Check sheet for the modelled part. Datum: model origin and axes. Units: mm. Face numbers are marked on the shaded views. A direction names the side the tool comes from. Round coordinates to 2 decimals unless told otherwise and drop trailing zeros. Write each loop counter-clockwise with the first axis right and the second up, starting at its lowest first coordinate (ties: lowest second). Pieces come first, ordered by that corner, then holes. Notation, with made-up numbers: (25, 56.5) -> (51, 56.5) arc R11 cw to (51, 60.5) -> close; hole circle Ø8 at (87, -11). An arc over 180 degrees is marked (long way). Write item = value, one per line.
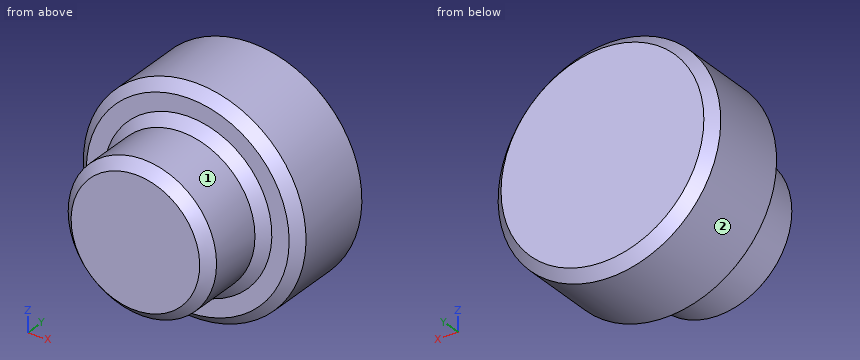
from build123d import *

# Parameters (mm, degrees)
SKETCH_1_R      = 3
EXTRUDE_1_DEPTH = 3
SKETCH_2_R      = 4.5
EXTRUDE_2_DEPTH = 4
CHAMFER_1_SIZE  = 0.4


with BuildPart() as part:
    # 草图1 → 凸台-拉伸1 (new body)
    with BuildSketch(Plane(origin=(0, 0, 0), x_dir=(1, 0, 0), z_dir=(0, 1, 0))):
        with Locations(Location((0, 0, 0), (0, 0, 270))):
            Circle(SKETCH_1_R)
    extrude(amount=EXTRUDE_1_DEPTH)

    # 草图2 → 凸台-拉伸2 (add)
    with BuildSketch(Plane(origin=(0, 3, 0), x_dir=(1, 0, 0), z_dir=(0, 1, 0))):
        with Locations(Location((0, 0, 0), (0, 0, 270))):
            Circle(SKETCH_2_R)
    extrude(amount=EXTRUDE_2_DEPTH)

    # 倒角1
    chamfer_1_edges = [part.edges().sort_by_distance(p)[0] for p in [
        (0, 0, -3),
        (0, 3, -3),
        (0, 3, -4.5),
        (0, 7, -4.5),
    ]]
    chamfer(chamfer_1_edges, length=CHAMFER_1_SIZE)


solid = part.part
(1) Sectioned sample at C-C on y = 4.5. Enter the section's corners in (x, z), then the cut area to 3 significant figures.
Worked answers:
outline = circle Ø9 at (0, 0)
area = 63.6 mm²
(2) Sectioned sample at D-D on y = 1.5. Enter the section's corners in (x, z).
Worked answers:
outline = circle Ø6 at (0, 0)
(3) Sectioned sample at A-A on x = 0. Enter the section's corners in (y, z).
Worked answers:
outline = (0, -2.6) -> (0.4, -3) -> (2.6, -3) -> (3, -3.4) -> (3, -4.1) -> (3.4, -4.5) -> (6.6, -4.5) -> (7, -4.1) -> (7, 4.1) -> (6.6, 4.5) -> (3.4, 4.5) -> (3, 4.1) -> (3, 3.4) -> (2.6, 3) -> (0.4, 3) -> (0, 2.6) -> close
(4) Sectioned sample at B-B on z = 0. Enter the section's corners in (x, y), then the cut area to 3 significant figures.
Worked answers:
outline = (-4.5, 3.4) -> (-4.1, 3) -> (-3.4, 3) -> (-3, 2.6) -> (-3, 0.4) -> (-2.6, 0) -> (2.6, 0) -> (3, 0.4) -> (3, 2.6) -> (3.4, 3) -> (4.1, 3) -> (4.5, 3.4) -> (4.5, 6.6) -> (4.1, 7) -> (-4.1, 7) -> (-4.5, 6.6) -> close
area = 53.7 mm²
(5) Go/stop test with a flat-tipped pin: P1, Ø1.5, axis at x = -3.5, z = 1, coming from the -Y side. Record where the tip stops, or that it passes through.
Worked answers:
P1 = 0.29
(6) Material ranges on L1, parallel to X at y = 1.5, z = -1.5; L2, parallel to Y at x = 3.25, z = -1.75; L3, parallel to X at y = 1, z = 0, recorded low to high. Write a range as [from, to].
Worked answers:
L1 = [-2.6, 2.6]
L2 = [3, 7]
L3 = [-3, 3]
(7) Access from +Z, -Z, +X, -X, +Y, -Y to the whole of each face (thin tool, end or side, straight path). Record for the marked faces 1 and 2.
Worked answers:
face_1 = -Y
face_2 = +Y, -Y
